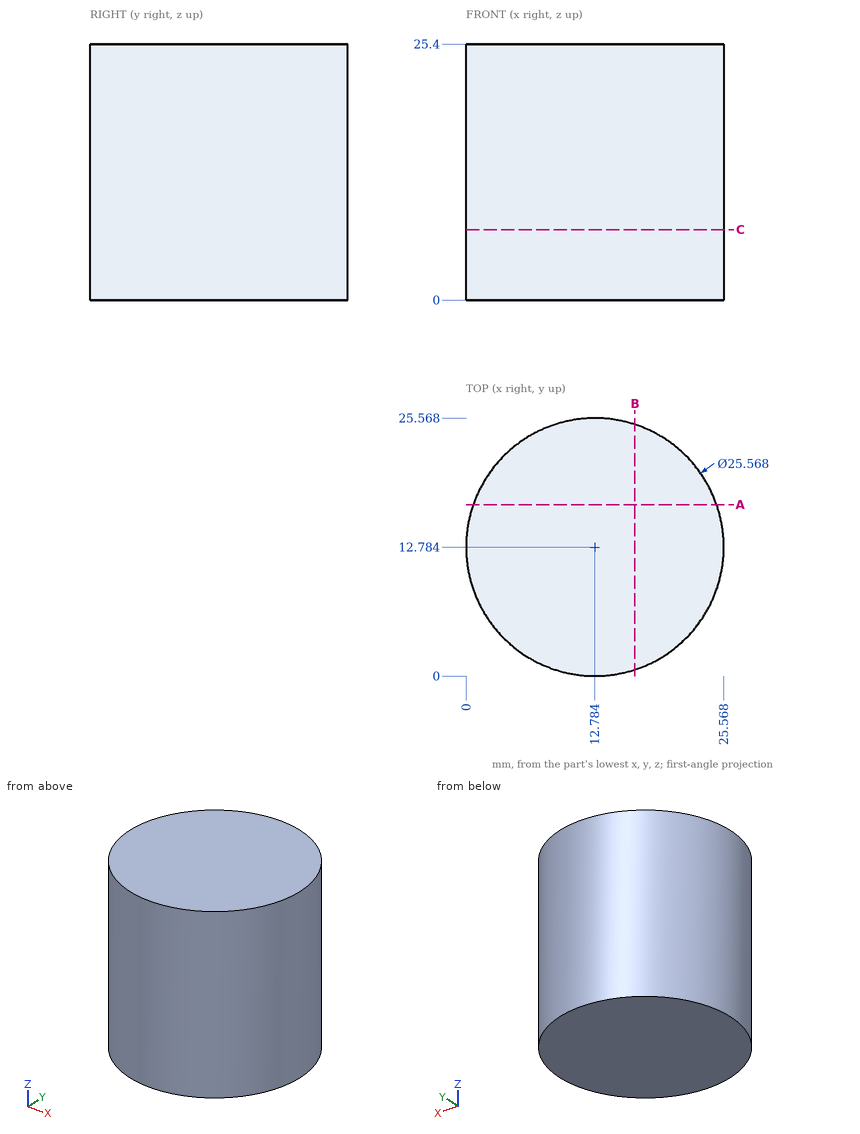
Drawing for the job (mm, zero at the part's lowest x, y, z). Coordinates: 2 decimals unless noted, no trailing zeros. Loops run counter-clockwise (first coordinate to the right, second up) from the corner with the lowest first, then second, coordinate; pieces in that order, holes last. Notation, with made-up numbers: (75.5, 55.25) - (121.5, 55.25) arc R31 ccw to (121.5, 81.25) - close; hole circle Ø3 at (74, 43.5). An arc over 180 degrees is marked (long way). Return JSON: item names as keys, results as strings.
1. Band-saw the part on B-B (x = 16.75). Give the cut face in (y, z).
Result:
{"outline": "(0.63, 0) - (24.94, 0) - (24.94, 25.4) - (0.63, 25.4) - close"}
2. Band-saw the part on C-C (z = 7). Give the cut face in (x, y), and give its area (3 significant figures).
Result:
{"outline": "circle Ø25.57 at (12.78, 12.78)", "area": "513 mm2"}
3. Drop flat-ended pins along their axis: pin 1 (3 mm diameter, centred on x = 4, z = 21.5, fed in from -Y); pin 2 (3 mm diameter, centred on y = 2.5, z = 9.5, fed in from -X) (1 decimal); pin 3 (3 mm diameter, centred on y = 14.5, z = 13, fed in from -X). Give the stop position or say it passes through.
Result:
{"pin 1": "stops at y = 2.28", "pin 2": "stops at x = 3.5", "pin 3": "stops at x = 0"}
4. Probe L1, parallel to X at y = 13, z = 20 (1 decimal); L2, parallel to X at y = 5.5, z = 8.75; L3, parallel to Y at x = 3, z = 4.5 (1 decimal). List the from-to ranges inside material, lowest first. Write a range as from..to.
Result:
{"L1": "x = 0..25.6", "L2": "x = 2.28..23.29", "L3": "y = 4.6..21"}
5. Band-saw the part on A-A (y = 17). Give the cut face in (x, z) (1 decimal), and give its area (3 significant figures).
Result:
{"outline": "(0.7, 0) - (24.9, 0) - (24.9, 25.4) - (0.7, 25.4) - close", "area": "613 mm2"}
